Design review of the part built by this model. Coordinates are the model's own, in mm. A direction names the side the tool comes from. Give positions to 0.01 mm unless a question says otherwise; leave off trailing zeros. Loops run counter-clockwise (first coordinate to the right, second up) from the corner with the lowest first, then second, coordinate; pieces in that order, holes last. Notation, with made-up numbers: M 89,-4 L 125,-4 A25 ccw 125,22 Z; hole C 55.25,47 d11. An arc over 180 degrees is marked long. Answer as CSV lines item,"result".
```python
from build123d import *

# Parameters (mm, degrees)
F1_W     = 32
F1_H     = 20
F2_DEPTH = 2
F3_W     = 2
F3_H     = 12
F3_W_2   = 22
F3_H_2   = 2
F4_DEPTH = 2
F5_W     = 2
F5_H     = 6
F6_DEPTH = 1


with BuildPart() as f2:
    # F1 (on Top) → F2 (new body)
    with BuildSketch(Plane.XY):
        Rectangle(F1_W, F1_H)
    extrude(amount=F2_DEPTH)

    # F3 (on face) → F4 (join)
    with BuildSketch(Plane.XY.offset(2)):
        with Locations((-13, 2)):
            Rectangle(F3_W, F3_H)
        with Locations((1, 7)):
            Rectangle(F3_W_2, F3_H_2)
        with Locations((13, -2)):
            Rectangle(F3_W, F3_H)
        with Locations((-1, -7)):
            Rectangle(F3_W_2, F3_H_2)
    extrude(amount=F4_DEPTH)

    # F5 (on face) → F6 (cut)
    with BuildSketch(Plane.XY.offset(2)):
        with Locations((-9, 1)):
            Rectangle(F5_W, F5_H)
        Polygon((-10, -2), (-10, -4), (10, -4), (10, -2), (8, -2), (-8, -2), align=None)
        with Locations((9, 1)):
            Rectangle(F5_W, F5_H)
    extrude(amount=-F6_DEPTH, mode=Mode.SUBTRACT)


solid = f2.part
```
1. To check wall thickness, follow L1, parallel to X at y = -1.25, z = 1.45; L2, parallel to X at y = -2, z = 3.15; L3, parallel to Y at x = -1, z = 1.8. State the ranges of each line that lie inside material, in increasing order. Write a range as [from, to].
Answer block:
L1,"[-16, -10], [-8, 8], [10, 16]"
L2,"[-14, -12], [12, 14]"
L3,"[-10, -4], [-2, 10]"
2. For P1, Ø2.5, axis at x = 4, y = 1, coming from the +Z side; P2, Ø1.6, axis at y = 2, z = 3, coming from the +X side; P3, Ø5, axis at x = 9.5, y = 1, coming from the -Z side; P4, Ø0.6, axis at x = -12.5, z = 3.5, coming from the +Y side, all flat-tipped, find the tip position at first contact; note any pin that passes through.
Answer block:
P1,"z = 2"
P2,"x = 14"
P3,"z = 0"
P4,"y = 8"
3. We need section A-A, the plane z = 3. Write out the cut boundary in (x, y).
Answer block:
outline,"M -14,-4 L -12,-4 L -12,8 L -14,8 Z; M -12,-8 L 10,-8 L 10,-6 L -12,-6 Z; M -10,6 L 12,6 L 12,8 L -10,8 Z; M 12,-8 L 14,-8 L 14,4 L 12,4 Z"
4. For faces 1 (the flat face through (-13, -4, 3)), 2 (the flat face through (12, -2, 3)), 3 (the flat face through (-12, 2, 3)), 4 (the flat face through (1, 6, 3)), 5 (the flat face through (-1, -6, 3)), list the 3-axis set-ups (+Z, -Z, +X, -X, +Y, -Y) from which the entire face can be reached by the end or side of a thin tool; tool diameter is ignored.
Answer block:
face 1,"+Z, -X, -Y"
face 2,"+Z, -Y"
face 3,"+Z, +Y"
face 4,"+Z, +X"
face 5,"+Z, -X"
5. We need section C-C, the plane y = -3.5. Write out the cut boundary in (x, z).
Answer block:
outline,"M -16,0 L 16,0 L 16,2 L 14,2 L 14,4 L 12,4 L 12,2 L 10,2 L 10,1 L -10,1 L -10,2 L -12,2 L -12,4 L -14,4 L -14,2 L -16,2 Z"
6. We need section B-B, the plane x = -9. Write out the cut boundary in (y, z).
Answer block:
outline,"M -10,0 L 10,0 L 10,2 L 8,2 L 8,4 L 6,4 L 6,2 L 4,2 L 4,1 L -4,1 L -4,2 L -6,2 L -6,4 L -8,4 L -8,2 L -10,2 Z"
7. The part is to be moulded in two halves that separate along Y. For faces 6 (the flat face through (-1, -7, 4)), 7 (the flat face through (-10, 0.1, 1.5)), 8 (the flat face through (13, 4, 3)), say which applies: pulls with the +Y half, pulls with the -Y half, needs draft (parallel to the pull), parting line crosses it, or undercut.
Answer block:
face 6,"needs draft"
face 7,"undercut"
face 8,"pulls with the +Y half"
8. We need section D-D, the plane y = -7.5. Write out the cut boundary in (x, z).
Answer block:
outline,"M -16,0 L 16,0 L 16,2 L 14,2 L 14,4 L 12,4 L 12,2 L 10,2 L 10,4 L -12,4 L -12,2 L -16,2 Z"
